Geometry check sheet. Reference: the model listing, model coordinates, mm. Coordinates: 2 decimals unless noted, no trailing zeros. Answer in a Markdown table with one row per item. Add a question column.
Q1. Section check A-A, the plane z = 318.5. Count the separate pieces of the cut face and the enclosed holes in it, and give its area (3 significant figures).
Q2. Thickness scan on line 1 (Y direction, x = -25, z = 1033.5); line 2 (Y direction, x = 15, z = 1344); line 3 (Y direction, x = -14, z = 300). Record the ranges inside material, lowest first.
Q3. Gauge pin test, flat end, axial feed: P1, Ø1.8, axis at x = 14, z = 774, coming from the +Y side. Record the tip position at first contact, or that the pin passes through.
```python
from build123d import *

# Parameters (mm, degrees)
F0_R     = 3
F0_R_2   = 2.5
F1_DEPTH = 1900
F2_R     = 2
F3_R     = 7


# Not quite as in the source:
# - a feature names something its author has since deleted; it is built from what else it names


with BuildPart() as f1:
    # F0 (on Top) → F1 (new body)
    with BuildSketch(Plane.XY):
        with BuildLine():
            Line((18.15, -30), (30, -30))
            Line((30, -30), (30, -18.15))
            Line((30, -18.15), (27.5, -18.15))
            Line((27.5, -18.15), (27.5, -20.15))
            Line((27.5, -20.15), (21.5477069044, -20.15))
            ThreePointArc((21.5477069044, -20.15), (19.5, -15), (21.5477069044, -9.85))
            Line((21.5477069044, -9.85), (27.5, -9.85))
            Line((27.5, -9.85), (27.5, -11.85))
            Line((27.5, -11.85), (30, -11.85))
            Line((30, -11.85), (30, 11.85))
            Line((30, 11.85), (27.5, 11.85))
            Line((27.5, 11.85), (27.5, 9.85))
            Line((27.5, 9.85), (21.5477069044, 9.85))
            ThreePointArc((21.5477069044, 9.85), (19.5, 15), (21.5477069044, 20.15))
            Line((21.5477069044, 20.15), (27.5, 20.15))
            Line((27.5, 20.15), (27.5, 18.15))
            Line((27.5, 18.15), (30, 18.15))
            Line((30, 18.15), (30, 30))
            Line((30, 30), (18.15, 30))
            Line((18.15, 30), (18.15, 27.5))
            Line((18.15, 27.5), (20.15, 27.5))
            Line((20.15, 27.5), (20.15, 21.5477069044))
            ThreePointArc((20.15, 21.5477069044), (15, 19.5), (9.85, 21.5477069044))
            Line((9.85, 21.5477069044), (9.85, 27.5))
            Line((9.85, 27.5), (11.85, 27.5))
            Line((11.85, 27.5), (11.85, 30))
            Line((11.85, 30), (-11.85, 30))
            Line((-11.85, 30), (-11.85, 27.5))
            Line((-11.85, 27.5), (-9.85, 27.5))
            Line((-9.85, 27.5), (-9.85, 21.5477069044))
            ThreePointArc((-9.85, 21.5477069044), (-15, 19.5), (-20.15, 21.5477069044))
            Line((-20.15, 21.5477069044), (-20.15, 27.5))
            Line((-20.15, 27.5), (-18.15, 27.5))
            Line((-18.15, 27.5), (-18.15, 30))
            Line((-18.15, 30), (-30, 30))
            Line((-30, 30), (-30, 18.15))
            Line((-30, 18.15), (-27.5, 18.15))
            Line((-27.5, 18.15), (-27.5, 20.15))
            Line((-27.5, 20.15), (-21.5477069044, 20.15))
            ThreePointArc((-21.5477069044, 20.15), (-19.5, 15), (-21.5477069044, 9.85))
            Line((-21.5477069044, 9.85), (-27.5, 9.85))
            Line((-27.5, 9.85), (-27.5, 11.85))
            Line((-27.5, 11.85), (-30, 11.85))
            Line((-30, 11.85), (-30, -11.85))
            Line((-30, -11.85), (-27.5, -11.85))
            Line((-27.5, -11.85), (-27.5, -9.85))
            Line((-27.5, -9.85), (-21.5477069044, -9.85))
            ThreePointArc((-21.5477069044, -9.85), (-19.5, -15), (-21.5477069044, -20.15))
            Line((-21.5477069044, -20.15), (-27.5, -20.15))
            Line((-27.5, -20.15), (-27.5, -18.15))
            Line((-27.5, -18.15), (-30, -18.15))
            Line((-30, -18.15), (-30, -30))
            Line((-30, -30), (-18.15, -30))
            Line((-18.15, -30), (-18.15, -27.5))
            Line((-18.15, -27.5), (-20.15, -27.5))
            Line((-20.15, -27.5), (-20.15, -21.5477069044))
            ThreePointArc((-20.15, -21.5477069044), (-15, -19.5), (-9.85, -21.5477069044))
            Line((-9.85, -21.5477069044), (-9.85, -27.5))
            Line((-9.85, -27.5), (-11.85, -27.5))
            Line((-11.85, -27.5), (-11.85, -30))
            Line((-11.85, -30), (11.85, -30))
            Line((11.85, -30), (11.85, -27.5))
            Line((11.85, -27.5), (9.85, -27.5))
            Line((9.85, -27.5), (9.85, -21.5477069044))
            ThreePointArc((9.85, -21.5477069044), (15, -19.5), (20.15, -21.5477069044))
            Line((20.15, -21.5477069044), (20.15, -27.5))
            Line((20.15, -27.5), (18.15, -27.5))
            Line((18.15, -27.5), (18.15, -30))
        make_face()
        with Locations((-25, -25)):
            Circle(F0_R, mode=Mode.SUBTRACT)
        with Locations((-15, -15)):
            Circle(F0_R_2, mode=Mode.SUBTRACT)
        with Locations((25, -25)):
            Circle(F0_R, mode=Mode.SUBTRACT)
        with Locations((15, -15)):
            Circle(F0_R_2, mode=Mode.SUBTRACT)
        with Locations((-25, 25)):
            Circle(F0_R, mode=Mode.SUBTRACT)
        with Locations((-15, 15)):
            Circle(F0_R_2, mode=Mode.SUBTRACT)
        Polygon((-7, 22), (-7, 27.5), (0, 27.5), (7, 27.5), (7, 22), (10, 16), (10, 10), (16, 10), (22, 7), (27.5, 7), (27.5, 0), (27.5, -7), (22, -7), (16, -10), (10, -10), (10, -16), (7, -22), (7, -27.5), (0, -27.5), (-7, -27.5), (-7, -22), (-10, -16), (-10, -10), (-16, -10), (-22, -7), (-27.5, -7), (-27.5, 0), (-27.5, 7), (-22, 7), (-16, 10), (-10, 10), (-10, 16), align=None, mode=Mode.SUBTRACT)
        with Locations((15, 15)):
            Circle(F0_R_2, mode=Mode.SUBTRACT)
        with Locations((25, 25)):
            Circle(F0_R, mode=Mode.SUBTRACT)
    extrude(amount=F1_DEPTH)

    # F2
    f2_edges = [f1.edges().sort_by_distance(p)[0] for p in [
        (-7, 27.5, 950),
        (7, 27.5, 950),
    ]]
    fillet(f2_edges, radius=F2_R)

    # F3
    f3_edges = [f1.edges().sort_by_distance(p)[0] for p in [
        (-10, 16, 950),
        (10, 16, 950),
    ]]
    fillet(f3_edges, radius=F3_R)


solid = f1.part
```
Calculated:
| question | item | result |
|---|---|---|
| 1 | separate pieces | 1 |
| 1 | enclosed holes | 9 |
| 1 | area | 1,080 mm² |
| 2 | line 1 | y = -30 to -28, -22 to -20.15, -9.85 to -7, 7 to 9.85, 20.15 to 22, 28 to 30 |
| 2 | line 2 | y = -19.5 to -17.5, -12.5 to -10, 10 to 12.5, 17.5 to 19.5 |
| 2 | line 3 | y = -19.57 to -17.29, -12.71 to -10, 10 to 12.71, 17.29 to 19.57 |
| 3 | P1 | stops at y = 19.74 |
